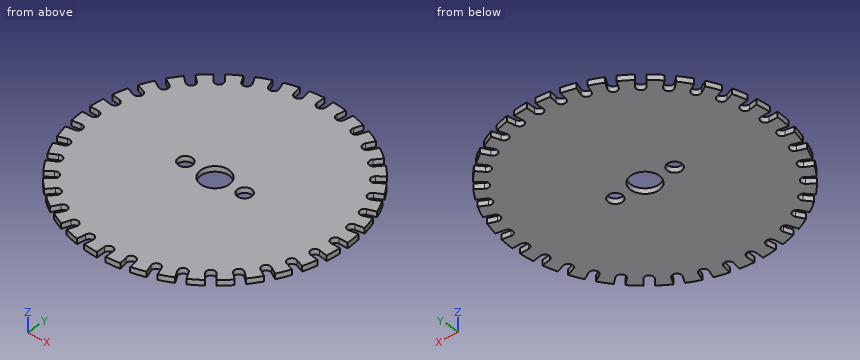
```python
from build123d import *

# Parameters (mm, degrees)
ESQUISSE1_R                  = 37
ESQUISSE1_R_2                = 4
ESQUISSE1_R_3                = 2
BOSS_EXTRU_1_DEPTH           = 1.5
ENL_V_MAT_EXTRU_1_DEPTH      = 53.347397261
R_P_TITION_CIRCULAIRE1_COUNT = 36


with BuildPart() as part:
    # Esquisse1 → Boss.-Extru.1 (new body)
    with BuildSketch(Plane.XY):
        Circle(ESQUISSE1_R)
        Circle(ESQUISSE1_R_2, mode=Mode.SUBTRACT)
        with Locations((8.5, 0)):
            Circle(ESQUISSE1_R_3, mode=Mode.SUBTRACT)
        with Locations((-8.5, 0)):
            Circle(ESQUISSE1_R_3, mode=Mode.SUBTRACT)
    extrude(amount=BOSS_EXTRU_1_DEPTH)

    # Esquisse2 → Enlèv. mat.-Extru.1 (cut, through all)
    with BuildSketch(Plane.XY.offset(1.5)):
        with BuildLine():
            Line((-40.577200577, 1.25), (-34.55, 1.25))
            ThreePointArc((-34.55, 1.25), (-33.3, 0), (-34.55, -1.25))
            Line((-34.55, -1.25), (-40.577200577, -1.25))
            ThreePointArc((-40.577200577, -1.25), (-41.827200577, 0), (-40.577200577, 1.25))
        make_face()
    enl_v_mat_extru_1 = extrude(amount=-ENL_V_MAT_EXTRU_1_DEPTH, mode=Mode.SUBTRACT)

    # Répétition circulaire1: Enlèv. mat.-Extru.1 ×36 about axis
    r_p_tition_circulaire1_axis = Axis((0, 0, 0), (0, 0, 1))
    for i in range(1, R_P_TITION_CIRCULAIRE1_COUNT):
        add(enl_v_mat_extru_1.rotate(r_p_tition_circulaire1_axis, i * 360 / R_P_TITION_CIRCULAIRE1_COUNT), mode=Mode.SUBTRACT)


solid = part.part
```
The listing builds one solid part. Answer for the finished solid, in the listing's coordinates (mm). Give positions to 0.01 mm unless a question says otherwise; leave off trailing zeros. Order: outer loops, then holes, each group sorted by start corner. A loop starts at its lowest first (then second) coordinate and runs counter-clockwise, first axis right, second up. Notation, with made-up numbers: (73.5, 51.5) -> (96.5, 51.5) arc R35 cw to (96.5, 86.5) -> close; hole circle Ø10 at (-24, 51.25). An arc over 180 degrees is marked (long way). One line per item, written item: value.
1) Find section D-D, the plane x = -9.5. Determine the outline of the cut face in (y, z), plus the area to 3 significant figures.
Reported:
outline: (-35.76, 0) -> (-1.73, 0) -> (-1.73, 1.5) -> (-35.76, 1.5) -> close; (1.73, 0) -> (35.76, 0) -> (35.76, 1.5) -> (1.73, 1.5) -> close
area: 102 mm^2
2) Find section B-B, the plane x = 8.5. Determine the outline of the cut face in (y, z), plus the area to 3 significant figures.
Reported:
outline: (-36.01, 0) -> (-2, 0) -> (-2, 1.5) -> (-36.01, 1.5) -> close; (2, 0) -> (36.01, 0) -> (36.01, 1.5) -> (2, 1.5) -> close
area: 102 mm^2
3) Find section A-A, the plane y = 0. Determine the outline of the cut face in (x, z), plus the area to 3 significant figures.
Reported:
outline: (-33.3, 0) -> (-10.5, 0) -> (-10.5, 1.5) -> (-33.3, 1.5) -> close; (-6.5, 0) -> (-4, 0) -> (-4, 1.5) -> (-6.5, 1.5) -> close; (4, 0) -> (6.5, 0) -> (6.5, 1.5) -> (4, 1.5) -> close; (10.5, 0) -> (33.3, 0) -> (33.3, 1.5) -> (10.5, 1.5) -> close
area: 75.9 mm^2
4) Find section C-C, the plane z = 0.6. Count the separate pieces of the cut face and the enclosed holes in it, plus the area to 3 significant figures.
Reported:
separate pieces: 1
enclosed holes: 3
area: 3,920 mm^2
5) Find the intervals of material crossed by line 1 (Y direction, x = 0, z = 0.4); line 2 (Y direction, x = 32.5, z = 0.75); line 3 (Y direction, x = 34.5, z = 1.15), in increasing order.
Reported:
line 1: y = -33.3 to -4, 4 to 33.3
line 2: y = -17.32 to -13.16, -10.57 to 10.57, 13.16 to 17.32
line 3: y = -11.23 to -7.35, -4.81 to -1.25, 1.25 to 4.81, 7.35 to 11.23
6) A flat-ended cylindrical pin translates along its axis: P1, Ø0.8, axis at y = 35.5, z = 1, coming from the +X side. Find the tip coordinate at first contact, or state that the pin passes through.
Reported:
P1: stops at x = 11.47
